Can you work these out from the model? Positions are in its coordinate system, mm. Face numbers are marked on the shaded views. A direction names the side the tool comes from. Round coordinates to 2 decimals unless told otherwise and drop trailing zeros. Loops run counter-clockwise (first coordinate to the right, second up) from the corner with the lowest first, then second, coordinate; pieces in that order, holes last.
from build123d import *

# Parameters (mm, degrees)
BOSS_EXTRUDE1_DEPTH = 11
FILLET2_R           = 2.5
SKETCH2_R           = 1.525
CUT_EXTRUDE1_DEPTH  = 22.05451258
FILLET3_R           = 5


with BuildPart() as part:
    # Sketch1 → Boss-Extrude1 (new body)
    with BuildSketch(Plane.XY):
        Polygon((-5.95, 0), (-5.95, 8), (5.95, 8), (5.95, 0), (5.95, -6.1), (-13.95, -6.1), (-13.95, -8.7), (7.95, -8.7), (7.95, 2.6), (7.95, 10.5), (-7.95, 10.5), (-7.95, 2.6), (-13.95, 2.6), (-13.95, 0), (-8.65875, 0), align=None)
    extrude(amount=BOSS_EXTRUDE1_DEPTH)

    # Fillet2
    fillet2_edges = [part.edges().sort_by_distance(p)[0] for p in [
        (-7.95, 10.5, 5.5),
        (7.95, 10.5, 5.5),
        (7.95, -8.7, 5.5),
    ]]
    fillet(fillet2_edges, radius=FILLET2_R)

    # Sketch2 → Cut-Extrude1 (cut, through all)
    with BuildSketch(Plane(origin=(0, 2.6, 0), x_dir=(1, 0, 0), z_dir=(0, 1, 0))):
        with Locations(Location((-10.95, -5.5, 0), (0, 0, 180))):
            Circle(SKETCH2_R)
    extrude(amount=-CUT_EXTRUDE1_DEPTH, mode=Mode.SUBTRACT)

    # Fillet3
    fillet3_edges = [part.edges().sort_by_distance(p)[0] for p in [
        (-13.95, 1.3, 0),
        (-13.95, -7.4, 0),
        (-13.95, -7.4, 11),
        (-13.95, 1.3, 11),
    ]]
    fillet(fillet3_edges, radius=FILLET3_R)


solid = part.part
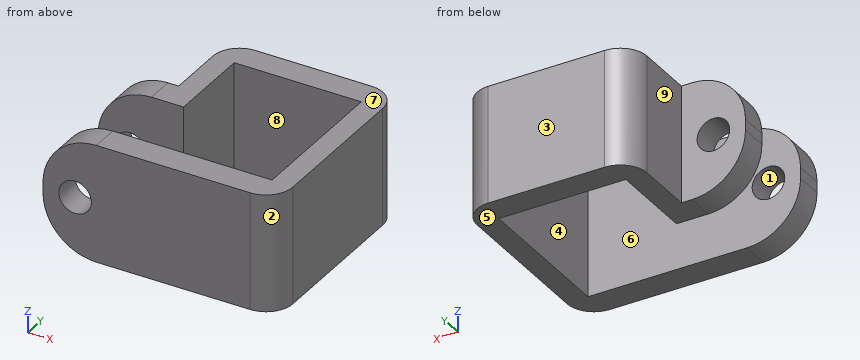
(1) If we section it at C-C, the plane x = -10.95: List the corners of the cut face in (y, z) for me (3 decimals), then the cut area to 3 significant figures.
Worked answers:
outline: (-8.7, 0.417) - (-6.1, 0.417) - (-6.1, 3.975) - (-8.7, 3.975) - close; (-8.7, 7.025) - (-6.1, 7.025) - (-6.1, 10.583) - (-8.7, 10.583) - close; (0, 0.417) - (2.6, 0.417) - (2.6, 3.975) - (0, 3.975) - close; (0, 7.025) - (2.6, 7.025) - (2.6, 10.583) - (0, 10.583) - close
area: 37.0 mm2
(2) If we section it at A-A, the plane x = -0.25: List the corners of the cut face in (y, z) for me, then the cut area to 3 significant figures.
Worked answers:
outline: (-8.7, 0) - (-6.1, 0) - (-6.1, 11) - (-8.7, 11) - close; (8, 0) - (10.5, 0) - (10.5, 11) - (8, 11) - close
area: 56.1 mm2
(3) If we mould it in two halves opening along Y, with no side actions, what happens to the marked faces 1, 2, 3 and 4? For each: released by +Y, released by -Y, zero draft, split by the parting line, or undercut.
Worked answers:
face 1: zero draft
face 2: released by -Y
face 3: released by +Y
face 4: undercut
(4) If we section it at B-B, the plane z = 5.5: List the corners of the cut face in (x, y) for me (3 decimals), then the cut area to 3 significant figures.
Worked answers:
outline: (-13.95, -8.7) - (-12.475, -8.7) - (-12.475, -6.1) - (-13.95, -6.1) - close; (-13.95, 0) - (-12.475, 0) - (-12.475, 2.6) - (-13.95, 2.6) - close; (-9.425, -8.7) - (5.45, -8.7) arc R2.5 ccw to (7.95, -6.2) - (7.95, 8) arc R2.5 ccw to (5.45, 10.5) - (-5.45, 10.5) arc R2.5 ccw to (-7.95, 8) - (-7.95, 2.6) - (-9.425, 2.6) - (-9.425, 0) - (-5.95, 0) - (-5.95, 8) - (5.95, 8) - (5.95, -6.1) - (-9.425, -6.1) - close
area: 137 mm2
(5) If I drill on line 1 (X direction, y = 6.25, z = 1.75); line 2 (Y direction, x = 2.5, z = 5.75); line 3 (Y direction, x = -9.75, z = 8.5), over which ranges is the centre line in solid material (lowest first)?
Worked answers:
line 1: x = -7.95 to -5.95, 5.95 to 7.95
line 2: y = -8.7 to -6.1, 8 to 10.5
line 3: y = -8.7 to -6.1, 0 to 2.6
(6) For the marked faces 5, 6, 7, 8 and 9, which set-ups out of +Z, -Z, +X, -X, +Y, -Y let a thin tool reach every point of the face, with its end or its side?
Worked answers:
face 5: -Z, +X, -X, +Y, -Y
face 6: +Z, -Z, -X
face 7: +Z, +X, -X, +Y, -Y
face 8: +Z, -Z
face 9: +Z, -Z, -X, +Y
(7) Will these pins go through, and if not, where does the flat tip stop? P1, Ø3.5, axis at x = -10.95, z = 5.5, coming from the +Y side; P2, Ø6, axis at y = -3.5, z = 1.5, coming from the -X side.
Worked answers:
P1: stops at y = 2.6
P2: stops at x = -13.53
(8) If we section it at D-D, the plane y = -4: List the corners of the cut face in (x, z) for me, then the cut area to 3 significant figures.
Worked answers:
outline: (5.95, 0) - (7.95, 0) - (7.95, 11) - (5.95, 11) - close
area: 22.0 mm2
